from build123d import *

# Parameters (mm, degrees)
BASE_FLANGE1_DEPTH                                = 1
HEM1_START                                        = -13.232002457
HEM1_DEPTH                                        = 26
CSK_FOR_M2_5_OVAL_HEAD_MACHINE_SCREW1_D           = 3.1
CSK_FOR_M2_5_OVAL_HEAD_MACHINE_SCREW1_DEPTH       = 4
CSK_FOR_M2_5_OVAL_HEAD_MACHINE_SCREW1_CSINK_D     = 5.5
CSK_FOR_M2_5_OVAL_HEAD_MACHINE_SCREW1_CSINK_ANGLE = 90
CSK_FOR_M2_5_OVAL_HEAD_MACHINE_SCREW1_TIP         = 0.931333959


# Read off the part's stored shape, not the designer's step: Hem1
# Sheet-metal steps are written as plain solids
with BuildPart() as part:
    # Sketch1 → Base-Flange1 (new body)
    with BuildSketch(Plane(origin=(0, 0, 0), x_dir=(1, 0, 0), z_dir=(0, 1, 0))):
        Polygon((6.794487322, 26.482002457), (-13.205512678, 26.482002457), (-13.205512678, -26.017997543), (6.794487322, -26.017997543), (6.794487322, -12.767997543), (10.794487322, -12.767997543), (10.794487322, 13.232002457), (6.794487322, 13.232002457), align=None)
    extrude(amount=-BASE_FLANGE1_DEPTH)

    # Hem1 outline → Hem1 (add)
    with BuildSketch(Plane.XY.offset(HEM1_START)):
        with BuildLine():
            Line((8.794487322, -3), (7.794487322, -3))
            ThreePointArc((7.794487322, -3), (12.915807666, -5.121320344), (10.794487322, 0))
            Line((10.794487322, 0), (10.794487322, -1))
            ThreePointArc((10.794487322, -1), (12.208700884, -4.414213562), (8.794487322, -3))
        make_face()
    extrude(amount=HEM1_DEPTH)

    # CSK for M2.5 Oval Head Machine Screw1
    with Locations(Plane(origin=(-5.205512678, -1, -19.982002457), x_dir=(0, 0, -1), z_dir=(0, -1, 0))):
        with Locations((0, 0), (-39.5, 0)):
            CounterSinkHole(CSK_FOR_M2_5_OVAL_HEAD_MACHINE_SCREW1_D / 2, CSK_FOR_M2_5_OVAL_HEAD_MACHINE_SCREW1_CSINK_D / 2, depth=CSK_FOR_M2_5_OVAL_HEAD_MACHINE_SCREW1_DEPTH, counter_sink_angle=CSK_FOR_M2_5_OVAL_HEAD_MACHINE_SCREW1_CSINK_ANGLE)
            with Locations((0, 0, -(CSK_FOR_M2_5_OVAL_HEAD_MACHINE_SCREW1_DEPTH + CSK_FOR_M2_5_OVAL_HEAD_MACHINE_SCREW1_TIP / 2))):  # 118° drill point
                Cone(0, CSK_FOR_M2_5_OVAL_HEAD_MACHINE_SCREW1_D / 2, CSK_FOR_M2_5_OVAL_HEAD_MACHINE_SCREW1_TIP, mode=Mode.SUBTRACT)


solid = part.part
Could you check a few things on this model? Use its own coordinates, in mm. A direction names the side the tool comes from. Give positions to 0.01 mm unless a question says otherwise; leave off trailing zeros. Order: outer loops, then holes, each group sorted by start corner. A loop starts at its lowest first (then second) coordinate and runs counter-clockwise, first axis right, second up.
1. Suppose I cut it at A-A (y = -3.5). List the corners of the cut face in (x, z) for me, plus the area to 3 significant figures.
2. Suppose I cut it at B-B (z = 7). List the corners of the cut face in (x, y) for me, plus the area to 3 significant figures.
3. Suppose I cut it at D-D (z = -16.5). List the corners of the cut face in (x, y) for me, plus the area to 3 significant figures.
4. I need wall thicknesses on L1, parallel to X at y = -4.25, z = -5.5; L2, parallel to Y at x = -2, z = -21; L3, parallel to Z at x = 11.25, y = -1. Which ranges of each line are inside material? Lowest first, please.
5. Suppose I cut it at C-C (x = 0.5). List the corners of the cut face in (y, z) for me.
6. Will these pins go through, and if not, where does the flat tip stop? P1, Ø2, axis at x = 8, z = -10.5, coming from the -Y side; P2, Ø12, axis at x = 4.5, z = -3.5, coming from the -Y side; P3, Ø1.5, axis at y = -2.5, z = 14.5, coming from the +X side; P4, Ø0.8, axis at y = -0.5, z = -17, coming from the +X side.
7. For faces 1 (the flat face through (6.794, -0.5, -19.8)), 2 (the flat face through (8, -3, 0)), 3 (the flat face through (8.7, -3.6, 12.768)), which set-ups out of +Z, -Z, +X, -X, +Y, -Y let a thin tool reach every point of the face, with its end or its side?
Solved:
1. outline: (7.84, -13.23) - (8.86, -13.23) - (8.86, 12.77) - (7.84, 12.77) - close; (12.73, -13.23) - (13.75, -13.23) - (13.75, 12.77) - (12.73, 12.77) - close
1. area: 53.1 mm2
2. outline: (-13.21, -1) - (10.79, -1) arc R2 cw (long way) to (8.79, -3) - (7.79, -3) arc R3 ccw (long way) to (10.79, 0) - (-13.21, 0) - close
2. area: 35.8 mm2
3. outline: (-13.21, -1) - (6.79, -1) - (6.79, 0) - (-13.21, 0) - close
3. area: 20.0 mm2
4. L1: x = 8.07 to 9.23, 12.36 to 13.52
4. L2: y = -1 to 0
4. L3: z = -13.23 to 12.77
5. outline: (-1, -26.48) - (0, -26.48) - (0, 26.02) - (-1, 26.02) - close
6. P1: stops at y = -5.4
6. P2: stops at y = -5.99
6. P3: passes through
6. P4: stops at x = 6.79
7. face 1: -Z, +X, +Y, -Y
7. face 2: +Z, -Z, -X
7. face 3: +Z, +X, +Y, -Y
